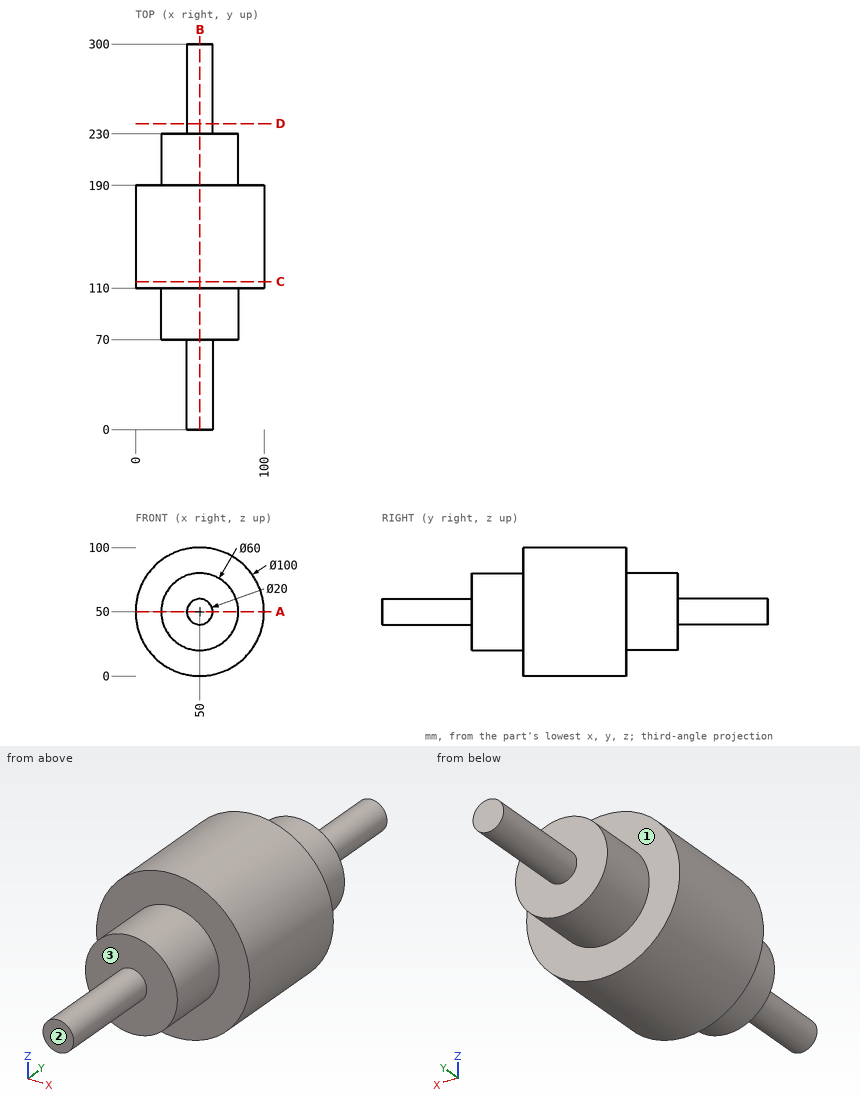
Geometry check sheet. Reference: drawing and pictorial views, mm from the part's lowest x, y, z. A direction names the side the tool comes from. Round coordinates to 2 decimals unless told otherwise and drop trailing zeros. Loops run counter-clockwise (first coordinate to the right, second up) from the corner with the lowest first, then second, coordinate; pieces in that order, holes last. Notation, with made-up numbers: (33, -29) - (89, -29) arc R21 ccw to (89, -14) - close; hole circle Ø7 at (17.25, -28). An arc over 180 degrees is marked (long way). Use a Markdown table: item, result.
Q1. Cross-section at C-C on y = 115. Record the cut outline in (x, z), plus the area to 3 significant figures.
Solutions:
| item | result |
|---|---|
| outline | circle Ø100 at (50, 50) |
| area | 7,850 mm2 |
Q2. Go/stop test with flat-tipped pins: P1, Ø6, axis at y = 33, z = 59, coming from the -X side; P2, Ø6, axis at y = 223.5, z = 20.5, coming from the +X side; P3, Ø10, axis at x = 29.5, z = 22, coming from the +Y side. Record where each tip stops, or that it passes through.
Solutions:
| item | result |
|---|---|
| P1 | stops at x = 42 |
| P2 | stops at x = 64.06 |
| P3 | stops at y = 230 |
Q3. Material ranges on line 1 (Y direction, x = 13, z = 23); line 2 (Y direction, x = 77.5, z = 39); line 3 (Z direction, x = 43, y = 85), recorded low to high.
Solutions:
| item | result |
|---|---|
| line 1 | y = 110 to 190 |
| line 2 | y = 70 to 230 |
| line 3 | z = 20.83 to 79.17 |
Q4. Cross-section at D-D on y = 238. Record the cut outline in (x, z), plus the area to 3 significant figures.
Solutions:
| item | result |
|---|---|
| outline | circle Ø20 at (50, 50) |
| area | 314 mm2 |
Q5. Cross-section at B-B on x = 50. Record the cut outline in (y, z).
Solutions:
| item | result |
|---|---|
| outline | (0, 40) - (70, 40) - (70, 20) - (110, 20) - (110, 0) - (190, 0) - (190, 20) - (230, 20) - (230, 40) - (300, 40) - (300, 60) - (230, 60) - (230, 80) - (190, 80) - (190, 100) - (110, 100) - (110, 80) - (70, 80) - (70, 60) - (0, 60) - close |
Q6. Cross-section at A-A on z = 50. Record the cut outline in (x, y).
Solutions:
| item | result |
|---|---|
| outline | (0, 110) - (20, 110) - (20, 70) - (40, 70) - (40, 0) - (60, 0) - (60, 70) - (80, 70) - (80, 110) - (100, 110) - (100, 190) - (80, 190) - (80, 230) - (60, 230) - (60, 300) - (40, 300) - (40, 230) - (20, 230) - (20, 190) - (0, 190) - close |
Q7. Access from +Z, -Z, +X, -X, +Y, -Y to the whole of each face (thin tool, end or side, straight path). Record for the marked faces 1, 2 and 3.
Solutions:
| item | result |
|---|---|
| face 1 | +Y |
| face 2 | +Z, -Z, +X, -X, -Y |
| face 3 | -Y |
